from build123d import *

# Parameters (mm, degrees)
SKETCH_1_W          = 12.4
SKETCH_1_H          = 5
EXTRUDE_1_DEPTH     = 10
SKETCH_2_W          = 1.2
SKETCH_2_H          = 0.6
SKETCH_2_W_2        = 1.6
CUT_EXTRUDE_1_DEPTH = 10


with BuildPart() as part:
    # 草图1 → 凸台-拉伸1 (new body)
    with BuildSketch(Plane.XY):
        Rectangle(SKETCH_1_W, SKETCH_1_H)
    extrude(amount=EXTRUDE_1_DEPTH)

    # 草图2 → 切除-拉伸1 (cut)
    with BuildSketch(Plane(origin=(0, 0, 0), x_dir=(-1, 0, 0), z_dir=(0, 0, -1))):
        with Locations((5.6, 2.2)):
            Rectangle(SKETCH_2_W, SKETCH_2_H)
        Polygon((5, 2.5), (4.8, 2.5), (4.8, 1.7), (6, 1.7), (6, 1), (5.160769515, 1), (6, -0.453589838), (6, -2.3), (-6, -2.3), (-6, -0.453589838), (-5.160769515, 1), (-6, 1), (-6, 1.7), (-4.4, 1.7), (-4.4, 2.5), (-4.6, 2.5), (-4.6, 1.9), (-6.2, 1.9), (-6.2, 0.8), (-5.507179677, 0.8), (-6.2, -0.4), (-6.2, -2.5), (6.2, -2.5), (6.2, -0.4), (5.507179677, 0.8), (6.2, 0.8), (6.2, 1.9), (5, 1.9), align=None)
        Polygon((6.2, -0.4), (6.2, 0.8), (5.507179677, 0.8), align=None)
        Polygon((-5.507179677, 0.8), (-6.2, 0.8), (-6.2, -0.4), align=None)
        with Locations((-5.4, 2.2)):
            Rectangle(SKETCH_2_W_2, SKETCH_2_H)
    extrude(amount=-CUT_EXTRUDE_1_DEPTH, mode=Mode.SUBTRACT)


solid = part.part
Geometry: final body of the model. Coordinates: model frame, mm. A direction names the side the tool comes from. Coordinates: 2 decimals unless noted, no trailing zeros. Order: outer loops, then holes, each group sorted by start corner. A loop starts at its lowest first (then second) coordinate and runs counter-clockwise, first axis right, second up.
(1) Section query C-C (y = 0.55). Return the cut outline in (x, z), plus the area to 3 significant figures.
(2) Section query A-A (z = 8.5). Return the cut outline in (x, y).
(3) Section query B-B (y = 2.1). Return the cut outline in (x, z).
(4) Draft query along Y for faces 1 (the face through (-5.6, 1, 4.9)), 2 (the face through (5, 1.7, 5)), 3 (the face through (-6, -1, 5)), 4 (the face through (5.6, 1, 4.9)). Return one class per face: pulls with the +Y half, pulls with the -Y half, needs draft (parallel to the pull), parting line crosses it, or undercut.
(5) Material intervals for probe 1 along X at (y, z) = (2.1, 6.5); probe 2 along Y at (x, z) = (5, 9); probe 3 along Y at (x, z) = (5.5, 4), sorted ascending.
(6) First-contact query: pin 1 (0.5 mm diameter, centred on x = 5.5, z = 4, fed in from +Y). Flat tip, straight axial feed; report the tip coordinate or a pass-through.
(7) Access query for faces 5 (the face through (5.59, 0.26, 4.93)), 6 (the face through (-5.575, 0.283, 4.93)), 7 (the face through (-5, 1.7, 5)). Directions: +Z, -Z, +X, -X, +Y, -Y. A direction counts if a zero-diameter tool reaches every point of the face in a straight line with its end or side. Return the directions, or none.
Solution:
1. outline: (-5.42, 0) - (5.42, 0) - (5.42, 10) - (-5.42, 10) - close
1. area: 108 mm2
2. outline: (-6, -2.3) - (6, -2.3) - (6, -0.45) - (5.16, 1) - (6, 1) - (6, 1.7) - (4.4, 1.7) - (4.4, 2.5) - (-4.8, 2.5) - (-4.8, 1.7) - (-6, 1.7) - (-6, 1) - (-5.16, 1) - (-6, -0.45) - close
3. outline: (-4.8, 0) - (4.4, 0) - (4.4, 10) - (-4.8, 10) - close
4. face 1: undercut
4. face 2: pulls with the +Y half
4. face 3: needs draft
4. face 4: undercut
5. probe 1: x = -4.8 to 4.4
5. probe 2: y = -2.3 to 1.7
5. probe 3: y = -2.3 to 0.41, 1 to 1.7
6. pin 1: stops at y = 1.7
7. face 5: +Z, -Z, +X
7. face 6: +Z, -Z, -X
7. face 7: +Z, -Z, -X, +Y
